Autodesk Inventor part; units mm, degrees
ref_plane "YZ Plane" through (0, 0, 0) normal (1, 0, 0) x (0, 1, 0)
ref_plane "XZ Plane" through (0, 0, 0) normal (0, 1, 0) x (-1, 0, 0)
ref_plane "XY Plane" through (0, 0, 0) normal (0, 0, 1) x (1, 0, 0)
sketch "Esboço3" plane through (0, 0, 0) normal (0, 0, 1) x (1, 0, 0)
  arc A0 (-23, -30) -> (-15, -38) centre (-15, -30) ccw
  line L0 (-23, -30) -> (-23, 30)
  arc A1 (-15, 38) -> (-23, 30) centre (-15, 30) ccw
  line L1 (-15, 38) -> (15, 38)
  arc A2 (23, 30) -> (15, 38) centre (15, 30) ccw
  line L2 (23, 30) -> (23, -30)
  arc A3 (15, -38) -> (23, -30) centre (15, -30) ccw
  line L3 (15, -38) -> (-15, -38)
  arc A4 (-25, -30) -> (-15, -40) centre (-15, -30) ccw
  line L4 (-15, -40) -> (15, -40)
  arc A5 (15, -40) -> (25, -30) centre (15, -30) ccw
  line L5 (25, -30) -> (25, 30)
  arc A6 (25, 30) -> (15, 40) centre (15, 30) ccw
  line L6 (15, 40) -> (-15, 40)
  arc A7 (-15, 40) -> (-25, 30) centre (-15, 30) ccw
  line L7 (-25, 30) -> (-25, -30)
  line L8 (-4, 12) -> (-4, 32)
  line L9 (-4, 32) -> (4, 32)
  line L10 (4, 12) -> (4, 32)
  line L11 (4, 12) -> (-4, 12)
  line L12 (-0.5, 40) -> (0.5, 40)
  line L13 (0.5, 40) -> (0.5, 32)
  line L14 (0.5, 32) -> (-0.5, 32)
  line L15 (-0.5, 32) -> (-0.5, 40)
  point P0 (0, 0)
  point P1 (0.5, 36)
  point P2 (0, 32)
  point P3 (-0.5, 38)
  point P4 (0.5, 38)
  dimension "d2" = 1
  dimension "d3" = 0
  dimension "d4" = 3.5
extrude "Extrusão1" add sketch "Esboço3" along normal blind 5 contours L0 A1 L1 L15 L9 L8 L11 L10 L13 A2 L2 A3 L3 A0 | A0 L3 A3 L2 A2 L1 L13 L6 A6 L5 A5 L4 A4 L7 A7 L15 A1 L0
fillet "Arredondamento1" radius 2 9 edges at (-22.0711, 37.0711, 5) (-25, 0, 5) (-22.0711, -37.0711, 5) (0, -40, 5) (22.0711, -37.0711, 5) (25, 0, 5) (22.0711, 37.0711, 5) (7.75, 40, 5) (-7.75, 40, 5)
shell "Casca1" thickness 2 removed faces 1 at (1.3333, -22.6667, 0)
properties part number "Tampa"
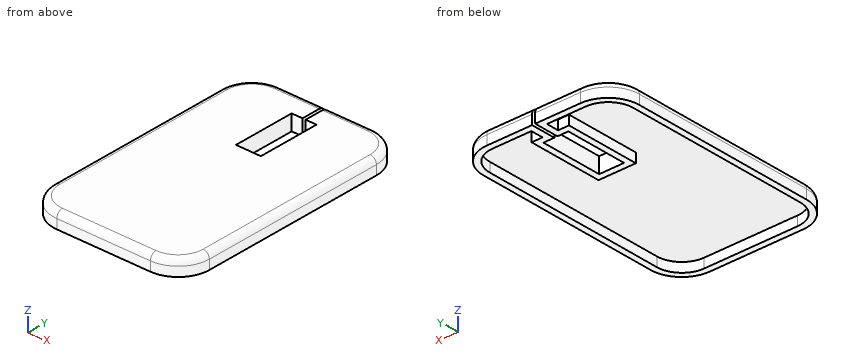
Can you work these out from the model? Positions are in its coordinate system, mm. Round coordinates to 2 decimals unless told otherwise and drop trailing zeros. Loops run counter-clockwise (first coordinate to the right, second up) from the corner with the lowest first, then second, coordinate; pieces in that order, holes last. Notation, with made-up numbers: (33, -35) - (57, -35) arc R20 cw to (57, 2) - close; hole circle Ø6 at (49.5, -10). An arc over 180 degrees is marked (long way). Answer in a Markdown table with one row per item. Add a question column.
Q1. I need wall thicknesses on L1, parallel to Y at x = -5.5, z = 2.4; L2, parallel to X at y = 25.5, z = 2.8; L3, parallel to Y at x = 2, z = 2.1. Which ranges of each line are inside material? Lowest first, please.
Q2. I want a section at C-C on x = 12. List the corners of the cut face in (y, z) for me.
Q3. I want a section at D-D on y = -26. List the corners of the cut face in (x, z) for me, and give its area (3 significant figures).
Q4. For pin 1 Ø12 at (x, y) = (-3, 0.5) entering from -Z; pin 2 Ø2.5 at (y, z) = (35.5, 2.5) entering from +X, each with a flat end and sliding along its axis, tell me the tip position at first contact or that it passes through.
Q5. I want a section at A-A on x = -1.5. List the corners of the cut face in (y, z) for me, and give its area (3 significant figures).
A:
| question | item | result |
|---|---|---|
| 1 | L1 | -40 to -38, 10 to 34, 38 to 40 |
| 1 | L2 | -25 to -23, -6 to -4, 4 to 6, 23 to 25 |
| 1 | L3 | -40 to -38, 10 to 12, 32 to 40 |
| 2 | outline | (-40, 0) - (-38, 0) - (-38, 3) - (38, 3) - (38, 0) - (40, 0) - (40, 3) arc R2 ccw to (38, 5) - (-38, 5) arc R2 ccw to (-40, 3) - close |
| 3 | outline | (-25, 0) - (-23, 0) - (-23, 3) - (23, 3) - (23, 0) - (25, 0) - (25, 3) arc R2 ccw to (23, 5) - (-23, 5) arc R2 ccw to (-25, 3) - close |
| 3 | area | 110 mm^2 |
| 4 | pin 1 | z = 3 |
| 4 | pin 2 | x = 24.05 |
| 5 | outline | (-40, 0) - (-38, 0) - (-38, 3) - (10, 3) - (10, 0) - (12, 0) - (12, 5) - (-38, 5) arc R2 ccw to (-40, 3) - close; (32, 0) - (40, 0) - (40, 3) arc R2 ccw to (38, 5) - (32, 5) - close |
| 5 | area | 154 mm^2 |
